The listing builds one solid part. Answer for the finished solid, in the listing's coordinates (mm). A direction names the side the tool comes from. Coordinates: 2 decimals unless noted, no trailing zeros. Order: outer loops, then holes, each group sorted by start corner. A loop starts at its lowest first (then second) coordinate and runs counter-clockwise, first axis right, second up. Notation, with made-up numbers: (-19.5, 58.25) - (21.5, 58.25) arc R26 ccw to (21.5, 78.25) - close; hole circle Ø11 at (10.5, -28). An arc over 180 degrees is marked (long way). Use a Markdown table: item, result. Add a question column.
Item 1: Flat-ended cylindrical pins translate along their axes: P1, Ø2.5, axis at x = 27.56, y = -21.04, coming from the -Z side (3 decimals); P2, Ø1, axis at y = -1, z = 1.5, coming from the +X side; P3, Ø0.5, axis at y = 6.5, z = 0.5, coming from the -X side. Find the tip coordinate at first contact, or state that the pin passes through.
Item 2: The part is cut by section C-C, the plane z = 1.1. State how many separate pieces and enclosed holes the cut face has, then the cut area to 3 significant figures.
Item 3: For faces 1 (the cylindrical face through (-34.016, -24.538, 0.913)), 2 (the cylindrical face through (33.93, 18.82, 0.91)), 3 (the cylindrical face through (36.13, -24.54, 0.91)), 4 (the flat face through (-26, -13.042, 1)), 5 (the cylindrical face through (21.826, -14.616, 0.913)), determine the directions among +Z, -Z, +X, -X, +Y, -Y from which every point of the face is accessible in a straight line to the end or side of a thin tool.
Item 4: The part is cut by section A-A, the plane x = 0.5. Give the vertices of the cut face in (y, z).
Item 5: The part is cut by section B-B, the plane y = -5. Give the vertices of the cut face in (x, z).
Item 6: Find the intervals of material crossed by line 1 along Y through (x, z) = (27.5, 0.1); line 2 along Y through (x, z) = (-25, 0.4); line 3 along X through (y, z) = (7, 0.9), in increasing order.
from build123d import *

# Parameters (mm, degrees)
F2_R     = 1.5
F2_W     = 30
F2_H     = 39
F3_DEPTH = 1.8
F5_R     = 5
F6_R     = 2


with BuildPart() as f3:
    # F2 (on Top) → F3 (new body)
    with BuildSketch(Plane.XY):
        Polygon((37.5577017069, 32.9581392366), (-35.4422982931, 32.9581392366), (-35.4422982931, 19.9581392366), (-16.6703661359, 19.9581392366), (-16.6703661359, -13.0418607634), (-35.4422982931, -13.0418607634), (-35.4422982931, -26.0418607634), (37.5577017069, -26.0418607634), (37.5577017069, -12.4774002814), (33.3296338641, -12.4774002814), (33.3296338641, 19.3936787546), (37.5577017069, 19.3936787546), align=None)
        with Locations((-30.4422982931, -21.0418607634)):
            Circle(F2_R, mode=Mode.SUBTRACT)
        with Locations((27.5577017069, -21.0418607634)):
            Circle(F2_R, mode=Mode.SUBTRACT)
        with Locations((8.3296338641, 3.4581392366)):
            Rectangle(F2_W, F2_H, mode=Mode.SUBTRACT)
        with Locations((-30.4422982931, 27.9581392366)):
            Circle(F2_R, mode=Mode.SUBTRACT)
        with Locations((27.5577017069, 27.9581392366)):
            Circle(F2_R, mode=Mode.SUBTRACT)
    extrude(amount=F3_DEPTH)

    # F5
    f5_edges = [f3.edges().sort_by_distance(p)[0] for p in [
        (-6.670366, 22.958139, 0.9),
        (-6.670366, -16.041861, 0.9),
        (23.329634, -16.041861, 0.9),
        (23.329634, 22.958139, 0.9),
        (-35.442298, -26.041861, 0.9),
        (37.557702, 32.958139, 0.9),
        (-35.442298, 32.958139, 0.9),
        (-16.670366, -13.041861, 0.9),
        (-16.670366, 19.958139, 0.9),
        (-35.442298, 19.958139, 0.9),
        (-35.442298, -13.041861, 0.9),
        (37.557702, -26.041861, 0.9),
    ]]
    fillet(f5_edges, radius=F5_R)

    # F6
    f6_edges = [f3.edges().sort_by_distance(p)[0] for p in [
        (37.557702, 19.393679, 0.9),
        (37.557702, -12.4774, 0.9),
        (33.329634, 19.393679, 0.9),
        (33.329634, -12.4774, 0.9),
    ]]
    fillet(f6_edges, radius=F6_R)


solid = f3.part
Solution:
| question | item | result |
|---|---|---|
| 1 | P1 | passes through |
| 1 | P2 | stops at x = 33.33 |
| 1 | P3 | stops at x = -16.67 |
| 2 | separate pieces | 1 |
| 2 | enclosed holes | 5 |
| 2 | area | 2,350 mm2 |
| 3 | face 1 | +Z, -Z, -X, -Y |
| 3 | face 2 | +Z, -Z, +X |
| 3 | face 3 | +Z, -Z, +X, -Y |
| 3 | face 4 | +Z, -Z, -X |
| 3 | face 5 | +Z, -Z |
| 4 | outline | (-26.04, 0) - (-16.04, 0) - (-16.04, 1.8) - (-26.04, 1.8) - close; (22.96, 0) - (32.96, 0) - (32.96, 1.8) - (22.96, 1.8) - close |
| 5 | outline | (-16.67, 0) - (-6.67, 0) - (-6.67, 1.8) - (-16.67, 1.8) - close; (23.33, 0) - (33.33, 0) - (33.33, 1.8) - (23.33, 1.8) - close |
| 6 | line 1 | y = -26.04 to -22.54, -19.54 to 26.46, 29.46 to 32.96 |
| 6 | line 2 | y = -26.04 to -13.04, 19.96 to 32.96 |
| 6 | line 3 | x = -16.67 to -6.67, 23.33 to 33.33 |
